Can you work these out from the drawing? Everything is in mm from the part's minimum corner. A direction names the side the tool comes from. Give positions to 0.01 mm unless a question says otherwise; leave off trailing zeros. Order: outer loops, then holes, each group sorted by start corner. A loop starts at its lowest first (then second) coordinate and runs counter-clockwise, first axis right, second up. Notation, with made-up numbers: M -14,52.25 L 23,52.25 A20 ccw 23,76.25 Z; hole C 47.5,23.5 d7. An arc over 180 degrees is marked long. Use a Markdown table: item, result. Add a question column.
Item 1: I'm going to push flat-ended pins straight in: pin 1 Ø15 at (y, z) = (21.5, 44.5) entering from +X; pin 2 Ø2.5 at (x, y) = (26.5, 27.5) entering from -Z; pin 3 Ø7.5 at (y, z) = (12, 2) entering from -X. Where does each tip first touch, or does it pass through?
Item 2: If I drill on L1, parallel to Y at x = 5.5, z = 69.5; L2, parallel to X at y = 33, z = 26.5; L3, parallel to Z at x = 7, y = 24.5, over which ranges is the centre line in solid material (lowest first)? Write a range as from..to.
Item 3: Suppose I cut it at A-A on y = 22. Write out the boundary of the cut face in (x, z), plus the area to 3 significant figures.
Item 4: Suppose I cut it at D-D on y = 17. Write out the boundary of the cut face in (x, z).
Item 5: For the marked faces 1, 2, 3, 4 and 5, which set-ups out of +Z, -Z, +X, -X, +Y, -Y let a thin tool reach every point of the face, with its end or its side?
Item 6: Suppose I cut it at C-C on z = 64.5. Write out the boundary of the cut face in (x, y), plus the area to 3 significant figures.
Item 7: Suppose I cut it at B-B on x = 29. Write out the boundary of the cut face in (y, z), plus the area to 3 significant figures.
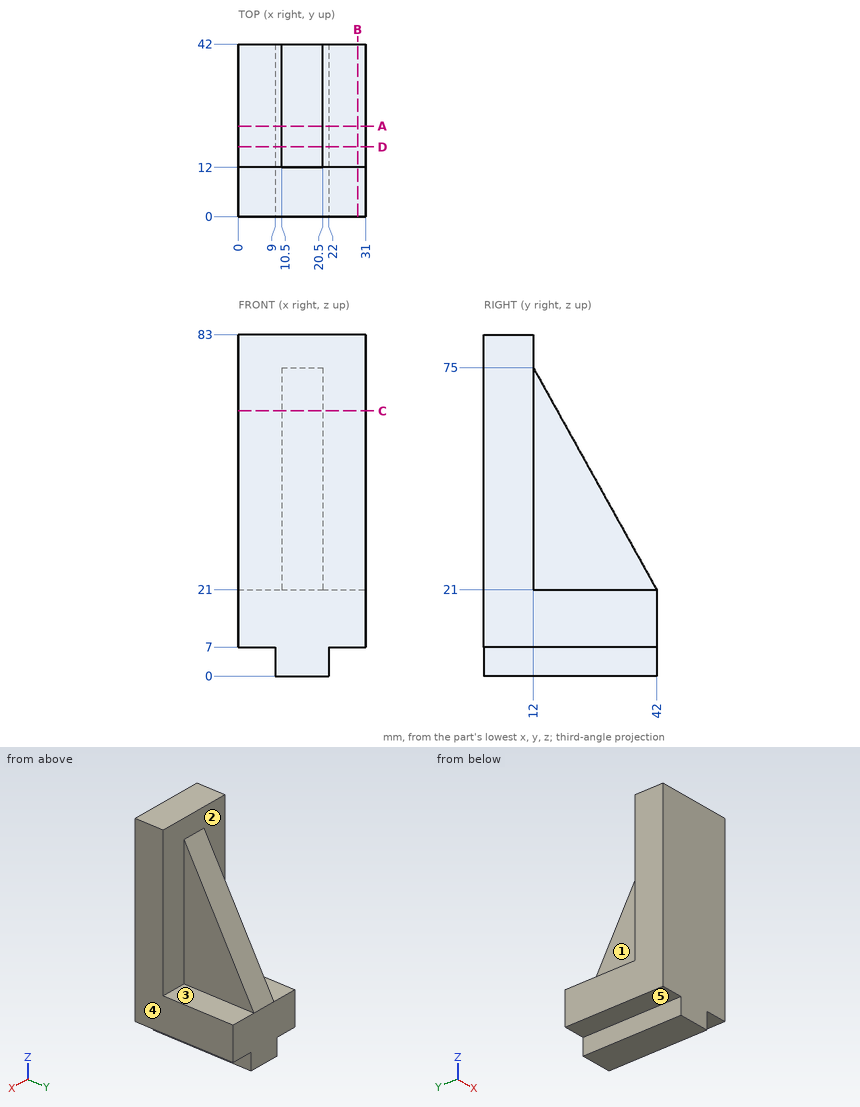
Findings below:
| question | item | result |
|---|---|---|
| 1 | pin 1 | stops at x = 20.5 |
| 1 | pin 2 | stops at z = 7 |
| 1 | pin 3 | stops at x = 9 |
| 2 | L1 | y = 0..12 |
| 2 | L2 | x = 10.5..20.5 |
| 2 | L3 | z = 7..21 |
| 3 | outline | M 0,7 L 9,7 L 9,0 L 22,0 L 22,7 L 31,7 L 31,21 L 20.5,21 L 20.5,57 L 10.5,57 L 10.5,21 L 0,21 Z |
| 3 | area | 885 mm^2 |
| 4 | outline | M 0,7 L 9,7 L 9,0 L 22,0 L 22,7 L 31,7 L 31,21 L 20.5,21 L 20.5,66 L 10.5,66 L 10.5,21 L 0,21 Z |
| 5 | face 1 | +Z, -X, +Y |
| 5 | face 2 | +Z, +Y |
| 5 | face 3 | +Z, +X, +Y |
| 5 | face 4 | +Z, -Z, +X, +Y, -Y |
| 5 | face 5 | -Z, -X, +Y, -Y |
| 6 | outline | M 0,0 L 31,0 L 31,12 L 20.5,12 L 20.5,17.83 L 10.5,17.83 L 10.5,12 L 0,12 Z |
| 6 | area | 430 mm^2 |
| 7 | outline | M 0,7 L 42,7 L 42,21 L 12,21 L 12,83 L 0,83 Z |
| 7 | area | 1,330 mm^2 |
